from build123d import *

# Parameters (mm, degrees)
F1_DEPTH = 5
F5_DEPTH = 3
F6_DEPTH = 3.2
F7_DEPTH = 7


with BuildPart() as f1:
    # F0 (on Top) → F1 (new body)
    with BuildSketch(Plane.XY):
        with BuildLine():
            Line((-2, 7.228416), (-2, 8.518363))
            ThreePointArc((-2, 8.518363), (0, -8.75), (2, 8.518363))
            Line((2, 8.518363), (2, 7.228416))
            ThreePointArc((2, 7.228416), (5.968668, 4.541476), (7.5, 0))
            ThreePointArc((7.5, 0), (-4.541476, -5.968668), (-2, 7.228416))
        make_face()
        with BuildLine():
            Line((-2, 8.518363), (-2, 10.816654))
            ThreePointArc((-2, 10.816654), (0, -11), (2, 10.816654))
            Line((2, 10.816654), (2, 8.518363))
            ThreePointArc((2, 8.518363), (0, -8.75), (-2, 8.518363))
        make_face()
        with BuildLine():
            Line((-2, 0), (-2, 7.228416))
            ThreePointArc((-2, 7.228416), (-4.541476, -5.968668), (7.5, 0))
            ThreePointArc((7.5, 0), (5.968668, 4.541476), (2, 7.228416))
            Line((2, 7.228416), (2, 0))
            ThreePointArc((2, 0), (0, -2), (-2, 0))
        make_face()
    extrude(amount=F1_DEPTH)

    # F1_face (on face) → F4 section 0
    with BuildSketch(Plane(origin=(0, -0.708891, 5), x_dir=(1, 0, 0), z_dir=(0, 0, 1))):
        with BuildLine():
            Line((-2, 0.708891), (-2, 11.525545))
            ThreePointArc((-2, 11.525545), (0, -10.291109), (2, 11.525545))
            Line((2, 11.525545), (2, 0.708891))
            ThreePointArc((2, 0.708891), (0, -1.291109), (-2, 0.708891))
        make_face()
    # F3 (on offset) → F4 section 1
    with BuildSketch(Plane.XY.offset(12)):
        with BuildLine():
            ThreePointArc((2, 3.172144), (0, -3.75), (-2, 3.172144))
            Line((-2, 3.172144), (-2, 4.582576))
            ThreePointArc((-2, 4.582576), (0, -5), (2, 4.582576))
            Line((2, 4.582576), (2, 3.172144))
        make_face()
    loft()

    # F0 (on Top) → F5 (cut)
    with BuildSketch(Plane.XY):
        with BuildLine():
            Line((-2, 8.518363), (-2, 10.816654))
            ThreePointArc((-2, 10.816654), (0, -11), (2, 10.816654))
            Line((2, 10.816654), (2, 8.518363))
            ThreePointArc((2, 8.518363), (0, -8.75), (-2, 8.518363))
        make_face()
    extrude(amount=F5_DEPTH, mode=Mode.SUBTRACT)

    # F3 (on offset) → F6 (cut)
    with BuildSketch(Plane.XY.offset(12)):
        with BuildLine():
            ThreePointArc((2, 0), (0, -2), (-2, 0))
            Line((-2, 0), (-2, 3.172144))
            ThreePointArc((-2, 3.172144), (0, -3.75), (2, 3.172144))
            Line((2, 3.172144), (2, 0))
        make_face()
    extrude(amount=-F6_DEPTH, mode=Mode.SUBTRACT)

    # F0 (on Top) → F7 (cut)
    with BuildSketch(Plane.XY):
        with BuildLine():
            Line((-2, 0), (-2, 7.228416))
            ThreePointArc((-2, 7.228416), (-4.541476, -5.968668), (7.5, 0))
            ThreePointArc((7.5, 0), (5.968668, 4.541476), (2, 7.228416))
            Line((2, 7.228416), (2, 0))
            ThreePointArc((2, 0), (0, -2), (-2, 0))
        make_face()
    extrude(amount=F7_DEPTH, mode=Mode.SUBTRACT)


solid = f1.part
Geometry: final body of the model. Coordinates: model frame, mm. A direction names the side the tool comes from. Coordinates: 2 decimals unless noted, no trailing zeros. Order: outer loops, then holes, each group sorted by start corner. A loop starts at its lowest first (then second) coordinate and runs counter-clockwise, first axis right, second up.
(1) Material intervals for probe 1 along X at (y, z) = (0, 10.3); probe 2 along Z at (x, y) = (-4.5, 1); probe 3 along X at (y, z) = (4.5, 2.25), sorted ascending.
(2) Draft query along X for faces 5 (the face through (0, -11, 4)), 6 (the face through (0, -8, 0)), 7 (the face through (-2, 7, 8)). Return one class per face: pulls with the +X half, pulls with the -X half, needs draft (parallel to the pull), parting line crosses it, or undercut.
(3) Section query A-A (z = 2). Return the cut outline in (x, y).
(4) Section query B-B (z = 3.5). Return the cut outline in (x, y).
(5) First-contact query: pin 1 (4 mm diameter, centred on y = -3, z = 8.5, fed in from +X); pin 2 (4 mm diameter, centred on y = 7, z = 6.5, fed in from +X); pin 3 (1 mm diameter, centred on x = 4, y = 8.5, fed in from +Z). Flat tips, straight axial feed; report the tip coordinate or a pass-through.
(6) Access query for faces 1 (the face through (1, -4, 12)), 2 (the face through (0, -3, 7)), 3 (the face through (2, 7, 8)), 4 (the face through (-1, -3, 8.8)). Directions: +Z, -Z, +X, -X, +Y, -Y. A direction counts if a zero-diameter tool reaches every point of the face in a straight line with its end or side. Return the directions, or none.
Solution:
1. probe 1: x = -6.44 to -3.75, 3.75 to 6.44
1. probe 2: z = 7 to 12
1. probe 3: x = -7.5 to -6, 6 to 7.5
2. face 5: parting line crosses it
2. face 6: needs draft
2. face 7: undercut
3. outline: (-2, 7.23) - (-2, 8.52) arc R8.75 ccw (long way) to (2, 8.52) - (2, 7.23) arc R7.5 cw (long way) to start
4. outline: (-2, 7.23) - (-2, 10.82) arc R11 ccw (long way) to (2, 10.82) - (2, 7.23) arc R7.5 cw (long way) to start
5. pin 1: stops at x = 9.33
5. pin 2: stops at x = 9.42
5. pin 3: stops at z = 7.42
6. face 1: +Z, +X, -X, +Y, -Y
6. face 2: -Z
6. face 3: +Z, -Z, +Y
6. face 4: +Z
